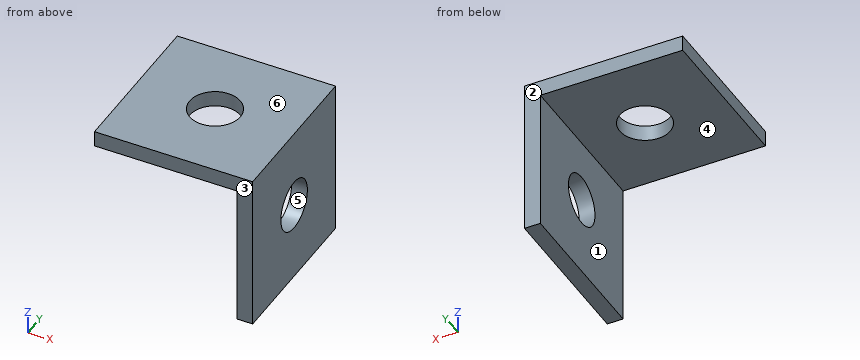
Autodesk Inventor part; units mm, degrees
ref_plane "YZ Plane" through (0, 0, 0) normal (1, 0, 0) x (0, 1, 0)
ref_plane "XZ Plane" through (0, 0, 0) normal (0, 1, 0) x (-1, 0, 0)
ref_plane "XY Plane" through (0, 0, 0) normal (0, 0, 1) x (1, 0, 0)
sketch "Sketch1" plane through (0, 0, 0) normal (0, 1, 0) x (-1, 0, 0)
  line L0 (0.8918, 0) -> (0, 0)
  line L1 (0, 0) -> (0, -10)
  line L2 (0, 0) -> (10, 0)
  line L3 (10, 0) -> (10, -1)
  line L4 (10, -1) -> (1, -1)
  line L5 (1, -1) -> (1, -10)
  line L6 (1, -10) -> (0, -10)
  dimension "d1" = 10
  dimension "d2" = 10
  dimension "d3" = 1
  dimension "d4" = 9
  dimension "d5" = 9
extrude "Extrusion1" add sketch "Sketch1" along normal blind 10
sketch "Sketch2" plane through (-10, 0, 0) normal (0, 0, 1) x (1, 0, 0)
  line L0 (-6.0649, 5) -> (16.1228, 5) construction
  line L1 (5, 14.125) -> (5, -1.5964) construction
  line L2 (0, 10) -> (10, 10) construction
  line L3 (10, 0) -> (10, 10) construction
  point P0 (5, 10)
  point P1 (10, 5)
  point P2 (5, 5)
hole "Hole1" at (-5, 5, 0) direction (0, 0, -1) diameter 3.2 end through all
sketch "Sketch3" plane through (0, 0, 0) normal (1, 0, 0) x (0, 0, -1)
  line L0 (5, 14.0037) -> (5, -2.6876)
  line L1 (-5.0316, 5) -> (14.0442, 5)
  line L2 (0, 10) -> (10, 10)
  line L3 (10, 0) -> (10, 10)
  point P0 (0, 0)
  point P1 (5, 10)
  point P2 (10, 5)
  point P3 (5, 5)
hole "Hole2" at (0, 5, -5) direction (-1, 0, 0) diameter 3.2 end through all
properties part number "No Thrd Right Support Farnell1466881"
Can you work these out from the model? Positions are in its coordinate system, mm. Face numbers are marked on the shaded views. A direction names the side the tool comes from. Give positions to 0.01 mm unless a question says otherwise; leave off trailing zeros. Order: outer loops, then holes, each group sorted by start corner. A loop starts at its lowest first (then second) coordinate and runs counter-clockwise, first axis right, second up. Notation, with made-up numbers: M 23,-32 L 38,-32 A17 ccw 38,-1 Z; hole C 32,-31 d4. An arc over 180 degrees is marked long. Use a Markdown table: item, result. Add a question column.
Item 1: Suppose I cut it at A-A (z = -5). List the corners of the cut face in (x, y) for me, then the cut area to 3 significant figures.
Item 2: Will these pins go through, and if not, where does the flat tip stop? pin 1 (5 mm diameter, centred on y = 8, z = -3, fed in from +X); pin 2 (3 mm diameter, centred on y = 5, z = -5, fed in from +X).
Item 3: Suppose I cut it at D-D (y = 7). List the corners of the cut face in (x, z) for me.
Item 4: Suppose I cut it at B-B (x = -5). List the corners of the cut face in (y, z) for me, then the cut area to 3 significant figures.
Item 5: Suppose I cut it at C-C (y = 5). List the corners of the cut face in (x, z) for me, then the cut area to 3 significant figures.
Item 6: We'd pull the mould along Z, two halves only. Please class the marked faces 3, 4, 5 and 6: +Z half, -Z half, draft (parallel to the pull), parting line (faces both ways), or undercut.
Item 7: For the marked faces 1 and 2, which set-ups out of +Z, -Z, +X, -X, +Y, -Y let a thin tool reach every point of the face, with its end or its side?
Item 8: If I drill on L1, parallel to X at y = 5, z = -0.5; L2, parallel to Y at x = -0.7, z = -5; L3, parallel to X at y = 7.75, z = -8, over which ranges is the centre line in solid material (lowest first)? Write a range as [from, to].
Answer sheet:
| question | item | result |
|---|---|---|
| 1 | outline | M -1,0 L 0,0 L 0,3.4 L -1,3.4 Z; M -1,6.6 L 0,6.6 L 0,10 L -1,10 Z |
| 1 | area | 6.80 mm² |
| 2 | pin 1 | stops at x = 0 |
| 2 | pin 2 | passes through |
| 3 | outline | M -10,-1 L -1,-1 L -1,-10 L 0,-10 L 0,0 L -10,0 Z |
| 4 | outline | M 0,-1 L 3.4,-1 L 3.4,0 L 0,0 Z; M 6.6,-1 L 10,-1 L 10,0 L 6.6,0 Z |
| 4 | area | 6.80 mm² |
| 5 | outline | M -10,-1 L -6.6,-1 L -6.6,0 L -10,0 Z; M -3.4,-1 L -1,-1 L -1,-3.4 L 0,-3.4 L 0,0 L -3.4,0 Z; M -1,-10 L 0,-10 L 0,-6.6 L -1,-6.6 Z |
| 5 | area | 12.6 mm² |
| 6 | face 3 | draft |
| 6 | face 4 | -Z half |
| 6 | face 5 | undercut |
| 6 | face 6 | +Z half |
| 7 | face 1 | -Z, -X, +Y, -Y |
| 7 | face 2 | +Z, -Z, +X, -X, +Y |
| 8 | L1 | x = [-10, -6.6], [-3.4, 0] |
| 8 | L2 | y = [0, 3.4], [6.6, 10] |
| 8 | L3 | x = [-1, 0] |
